from build123d import *

# Parameters (mm, degrees)
F0_R     = 24
F1_DEPTH = 10
F2_R     = 23
F3_DEPTH = 10.001


with BuildPart() as f1:
    # F0 (on Top) → F1 (new body)
    with BuildSketch(Plane.XY):
        Circle(F0_R)
    extrude(amount=F1_DEPTH)

    # F2 (on face) → F3 (cut, through all)
    with BuildSketch(Plane.XY.offset(10)):
        Circle(F2_R)
    extrude(amount=-F3_DEPTH, mode=Mode.SUBTRACT)

    # F4 (on Front) → F5 (revolve)
    with BuildSketch(Plane.XZ):
        Polygon((-23, 10), (-31.011236, 25.47067), (-31.011236, 36.581965), (-33.011236, 36.581965), (-33.011236, 25.581965), (-24, 10), align=None)
    revolve(axis=Axis((0, 0, 10), (0, 0, 1)))


solid = f1.part
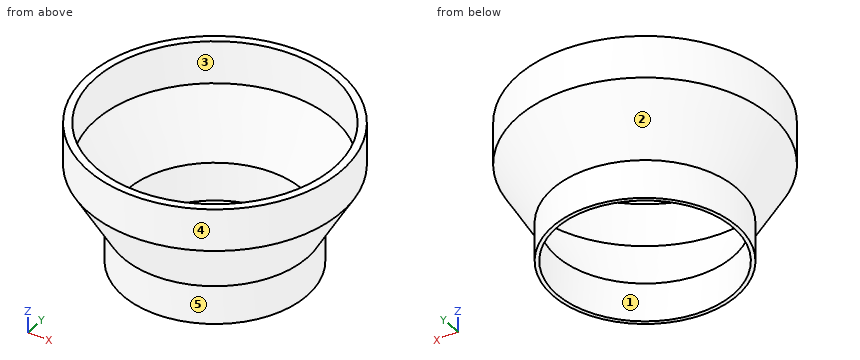
Can you work these out from the model? Positions are in its coordinate system, mm. Face numbers are marked on the shaded views. A direction names the side the tool comes from. Give positions to 0.01 mm unless a question says otherwise; leave off trailing zeros. Loops run counter-clockwise (first coordinate to the right, second up) from the corner with the lowest first, then second, coordinate; pieces in that order, holes last. Notation, with made-up numbers: (57, 87.25) - (69, 87.25) arc R25 ccw to (69, 114.25) - close; hole circle Ø8 at (68, -27). An arc over 180 degrees is marked (long way). Answer as a JSON object with one key per item and string values.
Q1. If I drill on L1, parallel to X at y = -0.5, z = 4; L2, parallel to X at y = 0, z = 30; L3, parallel to Y at x = 0, z = 7.75, over which ranges is the centre line in solid material (lowest first)?
Geometry says:
{"L1": "-23.99 to -22.99, 22.99 to 23.99", "L2": "-33.01 to -31.01, 31.01 to 33.01", "L3": "-24 to -23, 23 to 24"}
Q2. If we mould it in two halves opening along Y, with no side actions, what happens to the marked faces 1 and 2? For each: pulls with the +Y half, pulls with the -Y half, needs draft (parallel to the pull), parting line crosses it, or undercut.
Geometry says:
{"face 1": "undercut", "face 2": "parting line crosses it"}
Q3. Will these pins go through, and if not, where does the flat tip stop? P1, Ø1.5, axis at x = -8, z = 22.5, coming from the -Y side; P2, Ø6, axis at x = 18, z = 30, coming from the +Y side; P3, Ø3, axis at y = -14, z = 22.5, coming from the -X side.
Geometry says:
{"P1": "y = -30.67", "P2": "y = 29.41", "P3": "x = -29.11"}
Q4. Imagine slicing it at C-C on z = 34.5. Write out the boundary of the cut face in (x, y).
Geometry says:
{"outline": "circle Ø66.02 at (0, 0); hole circle Ø62.02 at (0, 0)"}
Q5. Imagine slicing it at A-A on x = 0. Write out the boundary of the cut face in (y, z).
Geometry says:
{"outline": "(-33.01, 25.58) - (-24, 10) - (-24, 0) - (-23, 0) - (-23, 10) - (-31.01, 25.47) - (-31.01, 36.58) - (-33.01, 36.58) - close; (23, 0) - (24, 0) - (24, 10) - (33.01, 25.58) - (33.01, 36.58) - (31.01, 36.58) - (31.01, 25.47) - (23, 10) - close"}
Q6. Imagine slicing it at D-D on z = 5. Write out the boundary of the cut face in (x, y).
Geometry says:
{"outline": "circle Ø48 at (0, 0); hole circle Ø46 at (0, 0)"}
Q7. Which directions (+Z, -Z, +X, -X, +Y, -Y) give clear straight access to the entire face, cutting with the end or side of a thin tool? Please do the marked faces 3, 4 and 5.
Geometry says:
{"face 3": "+Z", "face 4": "+Z, -Z", "face 5": "-Z"}
